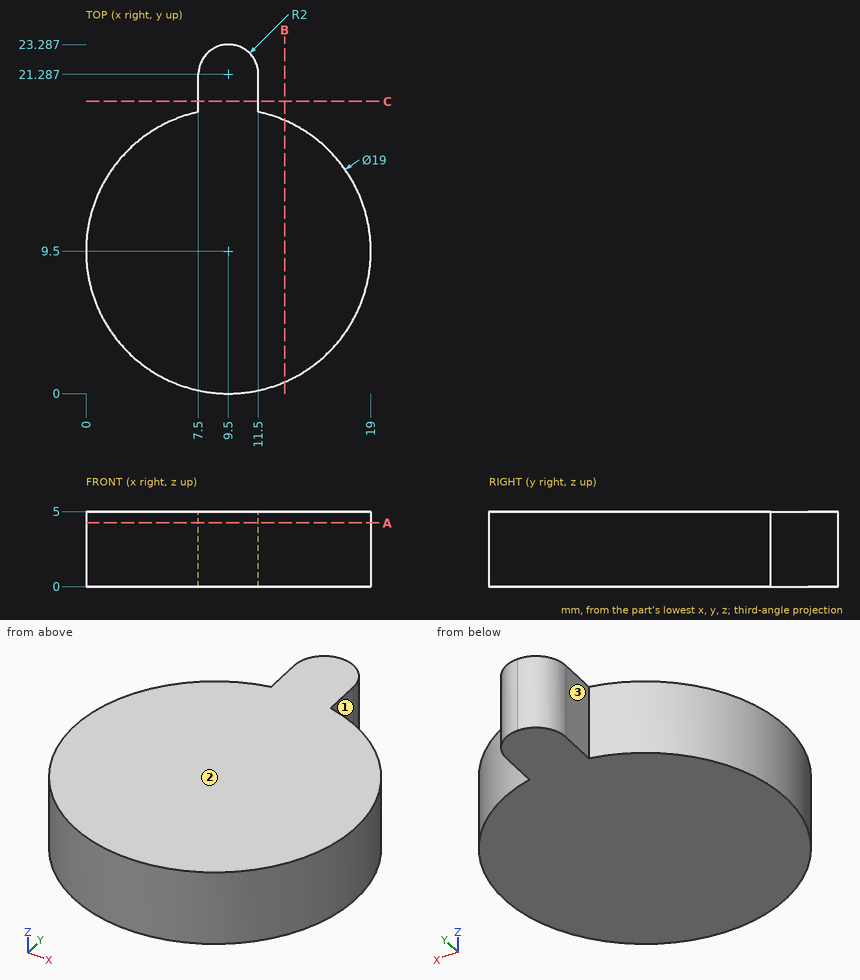
Answer from the drawing. Dimensions are ordinates in mm from the lowest x, y and z of the part. A direction names the side the tool comes from. Give positions to 0.01 mm unless a question says otherwise; leave off trailing zeros. Order: outer loops, then holes, each group sorted by start corner. A loop starts at its lowest first (then second) coordinate and runs counter-clockwise, first axis right, second up. Notation, with made-up numbers: (81, 16) -> (139, 16) arc R17 ccw to (139, 29) -> close; hole circle Ø2 at (-16, 68). An arc over 180 degrees is marked (long way). One line per item, written item: value.
Item 1: Find section B-B, the plane x = 13.25. Give the vertices of the cut face in (y, z).
Answer sheet:
outline: (0.77, 0) -> (18.23, 0) -> (18.23, 5) -> (0.77, 5) -> close
Item 2: Flat-ended cylindrical pins translate along their axes: P1, Ø1.5, axis at y = 11, z = 3.5, coming from the -X side; P2, Ø2, axis at y = 20, z = 2, coming from the -X side; P3, Ø1.5, axis at x = 12.5, z = 4, coming from the +Y side. Find the tip coordinate at first contact, or state that the pin passes through.
Answer sheet:
P1: x = 0.03
P2: x = 7.5
P3: y = 18.73
Item 3: Find section C-C, the plane y = 19.5. Give the vertices of the cut face in (x, z), plus the area to 3 significant figures.
Answer sheet:
outline: (7.5, 0) -> (11.5, 0) -> (11.5, 5) -> (7.5, 5) -> close
area: 20.0 mm²
Item 4: Find section A-A, the plane z = 4.25. Give the vertices of the cut face in (x, y), plus the area to 3 significant figures.
Answer sheet:
outline: (7.5, 18.79) arc R9.5 ccw (long way) to (11.5, 18.79) -> (11.5, 21.29) arc R2 ccw to (7.5, 21.29) -> close
area: 299 mm²
Item 5: Straight lines are drawn through the part: probe 1 along X at (y, z) = (9.5, 3.3); probe 2 along X at (y, z) = (19.5, 2.55); probe 3 along Y at (x, z) = (8.5, 1.3). For each, find the intervals that lie inside material, in ascending order.
Answer sheet:
probe 1: 0 to 19
probe 2: 7.5 to 11.5
probe 3: 0.05 to 23.02
Item 6: A tool of negligible diameter and unlimited length cuts with its end or side. For the marked faces 1, 2 and 3, from which of +Z, -Z, +X, -X, +Y, -Y can it reach the whole face along a straight path? Write none if from no direction.
Answer sheet:
face 1: +Z, -Z, +X, +Y
face 2: +Z, +X, -X, +Y, -Y
face 3: +Z, -Z, -X, +Y
